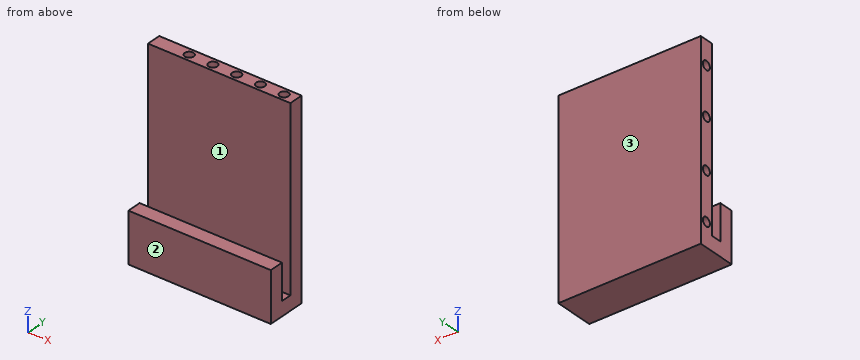
```python
from build123d import *

# Parameters (mm, degrees)
F1_DEPTH = 60
F3_DEPTH = 9
F4_R     = 1.875
F5_DEPTH = 10


with BuildPart() as f1:
    # F0 (on Right) → F1 (new body)
    with BuildSketch(Plane.YZ):
        Polygon((-0.522294, -6.121146), (-0.522294, -27.121146), (15.977706, -27.121146), (15.977706, 53.878854), (9.977706, 53.878854), (9.977706, -21.121146), (5.477706, -21.121146), (5.477706, -6.121146), align=None)
    extrude(amount=F1_DEPTH)

    # F2 (on face) → F3 (cut)
    with BuildSketch(Plane(origin=(0, 0, 0), x_dir=(0, -1, 0), z_dir=(-1, 0, 0))):
        with BuildLine():
            Line((-12.977706, 43.878854), (-12.977706, 45.753854))
            ThreePointArc((-12.977706, 45.753854), (-14.852706, 43.878854), (-12.977706, 42.003854))
            Line((-12.977706, 42.003854), (-12.977706, 43.878854))
        make_face()
        with BuildLine():
            ThreePointArc((-12.977706, 42.003854), (-11.651881, 42.553028), (-11.102706, 43.878854))
            ThreePointArc((-11.102706, 43.878854), (-11.651881, 45.204679), (-12.977706, 45.753854))
            Line((-12.977706, 45.753854), (-12.977706, 43.878854))
            Line((-12.977706, 43.878854), (-12.977706, 42.003854))
        make_face()
        with BuildLine():
            Line((-12.977706, 23.878854), (-12.977706, 25.753854))
            ThreePointArc((-12.977706, 25.753854), (-14.852706, 23.878854), (-12.977706, 22.003854))
            Line((-12.977706, 22.003854), (-12.977706, 23.878854))
        make_face()
        with BuildLine():
            ThreePointArc((-11.102706, 23.878854), (-11.651881, 25.204679), (-12.977706, 25.753854))
            Line((-12.977706, 25.753854), (-12.977706, 23.878854))
            Line((-12.977706, 23.878854), (-12.977706, 22.003854))
            ThreePointArc((-12.977706, 22.003854), (-11.651881, 22.553028), (-11.102706, 23.878854))
        make_face()
        with BuildLine():
            Line((-12.977706, 2.878854), (-12.977706, 4.753854))
            ThreePointArc((-12.977706, 4.753854), (-14.852706, 2.878854), (-12.977706, 1.003854))
            Line((-12.977706, 1.003854), (-12.977706, 2.878854))
        make_face()
        with BuildLine():
            ThreePointArc((-11.102706, 2.878854), (-11.651881, 4.204679), (-12.977706, 4.753854))
            Line((-12.977706, 4.753854), (-12.977706, 2.878854))
            Line((-12.977706, 2.878854), (-12.977706, 1.003854))
            ThreePointArc((-12.977706, 1.003854), (-11.651881, 1.553028), (-11.102706, 2.878854))
        make_face()
        with BuildLine():
            Line((-12.977706, -17.121146), (-12.977706, -15.246146))
            ThreePointArc((-12.977706, -15.246146), (-14.852706, -17.121146), (-12.977706, -18.996146))
            Line((-12.977706, -18.996146), (-12.977706, -17.121146))
        make_face()
        with BuildLine():
            ThreePointArc((-11.102706, -17.121146), (-11.651881, -15.795321), (-12.977706, -15.246146))
            Line((-12.977706, -15.246146), (-12.977706, -17.121146))
            Line((-12.977706, -17.121146), (-12.977706, -18.996146))
            ThreePointArc((-12.977706, -18.996146), (-11.651881, -18.446972), (-11.102706, -17.121146))
        make_face()
    extrude(amount=-F3_DEPTH, mode=Mode.SUBTRACT)

    # F4 (on face) → F5 (cut)
    with BuildSketch(Plane.XY.offset(53.878854)):
        with BuildLine():
            ThreePointArc((43.125, 12.977706), (45, 11.102706), (46.875, 12.977706))
            Line((46.875, 12.977706), (45, 12.977706))
            Line((45, 12.977706), (43.125, 12.977706))
        make_face()
        with BuildLine():
            ThreePointArc((56.875, 12.977706), (55, 14.852706), (53.125, 12.977706))
            Line((53.125, 12.977706), (55, 12.977706))
            Line((55, 12.977706), (56.875, 12.977706))
        make_face()
        with BuildLine():
            Line((55, 12.977706), (53.125, 12.977706))
            ThreePointArc((53.125, 12.977706), (55, 11.102706), (56.875, 12.977706))
            Line((56.875, 12.977706), (55, 12.977706))
        make_face()
        with BuildLine():
            Line((45, 12.977706), (46.875, 12.977706))
            ThreePointArc((46.875, 12.977706), (45, 14.852706), (43.125, 12.977706))
            Line((43.125, 12.977706), (45, 12.977706))
        make_face()
        with Locations((15, 12.977706)):
            Circle(F4_R)
        with BuildLine():
            ThreePointArc((23.125, 12.977706), (25, 11.102706), (26.875, 12.977706))
            Line((26.875, 12.977706), (25, 12.977706))
            Line((25, 12.977706), (23.125, 12.977706))
        make_face()
        with BuildLine():
            Line((25, 12.977706), (26.875, 12.977706))
            ThreePointArc((26.875, 12.977706), (25, 14.852706), (23.125, 12.977706))
            Line((23.125, 12.977706), (25, 12.977706))
        make_face()
        with BuildLine():
            ThreePointArc((33.125, 12.977706), (35, 11.102706), (36.875, 12.977706))
            Line((36.875, 12.977706), (35, 12.977706))
            Line((35, 12.977706), (33.125, 12.977706))
        make_face()
        with BuildLine():
            Line((35, 12.977706), (36.875, 12.977706))
            ThreePointArc((36.875, 12.977706), (35, 14.852706), (33.125, 12.977706))
            Line((33.125, 12.977706), (35, 12.977706))
        make_face()
    extrude(amount=-F5_DEPTH, mode=Mode.SUBTRACT)


solid = f1.part
```
Can you work these out from the model? Positions are in its coordinate system, mm. Face numbers are marked on the shaded views. Coordinates: 2 decimals unless noted, no trailing zeros. Loops run counter-clockwise (first coordinate to the right, second up) from the corner with the lowest first, then second, coordinate; pieces in that order, holes last. Notation, with made-up numbers: (76.5, 8.5) -> (96.5, 8.5) arc R16 ccw to (96.5, 26.5) -> close; hole circle Ø3 at (-3, -29.75). An arc over 180 degrees is marked (long way). Put each result on its own line as item: value. Start each with the question number.
Q1. I'm going to push flat-ended pins straight in: P1, Ø1.9, axis at x = 35, y = 13.5, coming from the +Z side; P2, Ø4, axis at x = 15, y = 14, coming from the +Z side; P3, Ø3, axis at x = 17.5, z = -2.5, coming from the -Y side; P4, Ø1.5, axis at x = 34, y = 5, coming from the +Z side. Where does each tip first touch, or does it pass through?
Q2. I want a section at A-A (x = 41). Write out the boundary of the cut face in (y, z).
Q3. Thinking about a two-plate mould opening in Y: for the marked faces 1, 2 and 3, which applies, pulls with the +Y half, pulls with the -Y half, needs draft (parallel to the pull), parting line crosses it, or undercut?
Q4. If I drill on line 1 (Y direction, x = 13.5, z = -9.5); line 2 (Y direction, x = 20, z = 21); line 3 (Y direction, x = 25, z = 46), over which ranges is the centre line in solid material (lowest first)? Write a range as [from, to].
Q5. I want a section at C-C (z = 16.5). Write out the boundary of the cut face in (x, y).
Q6. I want a section at D-D (x = 55). Write out the boundary of the cut face in (y, z).
Q7. I want a section at B-B (y = 0.5). Write out the boundary of the cut face in (x, z), plus the area to 3 significant figures.
Taken from the geometry:
1. P1: stops at z = 43.88
1. P2: stops at z = 53.88
1. P3: stops at y = 9.98
1. P4: stops at z = -6.12
2. outline: (-0.52, -27.12) -> (15.98, -27.12) -> (15.98, 53.88) -> (9.98, 53.88) -> (9.98, -21.12) -> (5.48, -21.12) -> (5.48, -6.12) -> (-0.52, -6.12) -> close
3. face 1: undercut
3. face 2: pulls with the -Y half
3. face 3: pulls with the +Y half
4. line 1: y = [-0.52, 5.48], [9.98, 15.98]
4. line 2: y = [9.98, 15.98]
4. line 3: y = [9.98, 11.1], [14.85, 15.98]
5. outline: (0, 9.98) -> (60, 9.98) -> (60, 15.98) -> (0, 15.98) -> close
6. outline: (-0.52, -27.12) -> (15.98, -27.12) -> (15.98, 53.88) -> (14.85, 53.88) -> (14.85, 43.88) -> (11.1, 43.88) -> (11.1, 53.88) -> (9.98, 53.88) -> (9.98, -21.12) -> (5.48, -21.12) -> (5.48, -6.12) -> (-0.52, -6.12) -> close
7. outline: (0, -27.12) -> (60, -27.12) -> (60, -6.12) -> (0, -6.12) -> close
7. area: 1,260 mm2
